from build123d import *

# Parameters (mm, degrees)
SKETCH1_W            = 105
SKETCH1_H            = 20
BOSS_EXTRUDE1_DEPTH  = 6.35
SKETCH3_W            = 23
SKETCH3_H            = 16
CUT_EXTRUDE1_DEPTH   = 54.819815124
SKETCH4_W            = 5
SKETCH4_H            = 12
CUT_EXTRUDE2_DEPTH   = 2
M2_CLEARANCE_HOLE1_D = 2


with BuildPart() as part:
    # Sketch1 → Boss-Extrude1 (new body)
    with BuildSketch(Plane(origin=(0, 0, 0), x_dir=(1, 0, 0), z_dir=(0, 1, 0))):
        Rectangle(SKETCH1_W, SKETCH1_H)
    extrude(amount=BOSS_EXTRUDE1_DEPTH)

    # Sketch3 → Cut-Extrude1 (cut, through all)
    with BuildSketch(Plane(origin=(0, 6.35, 0), x_dir=(1, 0, 0), z_dir=(0, 1, 0))):
        with Locations((-36, -2)):
            Rectangle(SKETCH3_W, SKETCH3_H)
        with Locations((36, 2)):
            Rectangle(SKETCH3_W, SKETCH3_H)
    extrude(amount=-CUT_EXTRUDE1_DEPTH, mode=Mode.SUBTRACT)

    # Sketch4 → Cut-Extrude2 (cut)
    with BuildSketch(Plane.XZ):
        with Locations((22, 0)):
            Rectangle(SKETCH4_W, SKETCH4_H)
        with Locations((50, 0)):
            Rectangle(SKETCH4_W, SKETCH4_H)
    extrude(amount=-CUT_EXTRUDE2_DEPTH, mode=Mode.SUBTRACT)

    # M2 Clearance Hole1 (through all)
    with Locations(Plane(origin=(0, 6.35, 0), x_dir=(1, 0, 0), z_dir=(0, 1, 0))):
        with Locations((50, 0), (-50, 0), (-22, 0), (22, 0)):
            Hole(M2_CLEARANCE_HOLE1_D / 2)


solid = part.part
Could you check a few things on this model? Use its own coordinates, in mm. A direction names the side the tool comes from. Round coordinates to 2 decimals unless told otherwise and drop trailing zeros. Write each loop counter-clockwise with the first axis right and the second up, starting at its lowest first coordinate (ties: lowest second). Pieces come first, ordered by that corner, then holes. Notation, with made-up numbers: (3, 57) - (19, 57) arc R29 ccw to (19, 81) - close; hole circle Ø4 at (39, 83). An arc over 180 degrees is marked (long way). Use a Markdown table: item, result.
Q1. For faces 1 (the flat face through (24.5, 4, -2)), 2 (the flat face through (-24.5, 3, 2)), 3 (the flat face through (48.85, 2, 0.08)), 4 (the flat face through (52.5, 4, 0)), which set-ups out of +Z, -Z, +X, -X, +Y, -Y let a thin tool reach every point of the face, with its end or its side?
Output values:
| item | result |
|---|---|
| face 1 | -Z, +Y, -Y |
| face 2 | +Z, +Y, -Y |
| face 3 | +X, -Y |
| face 4 | +Z, -Z, +X, +Y, -Y |
Q2. I want a section at B-B (x = 22). List the corners of the cut face in (y, z) for me, plus the area to 3 significant figures.
Output values:
| item | result |
|---|---|
| outline | (0, -10) - (6.35, -10) - (6.35, -1) - (2, -1) - (2, -6) - (0, -6) - close; (0, 6) - (2, 6) - (2, 1) - (6.35, 1) - (6.35, 10) - (0, 10) - close |
| area | 94.3 mm2 |
Q3. Thinking about a two-plate mould opening in X: for faces 5 (the flat face through (19.5, 1, 0)), 6 (the cylindrical face through (23, 4, 0)), 7 (the flat face through (-15, 3, -10)), which applies, released by +X, released by -X, zero draft, split by the parting line, or undercut?
Output values:
| item | result |
|---|---|
| face 5 | released by +X |
| face 6 | undercut |
| face 7 | zero draft |
Q4. I want a section at A-A (z = 0). Count the separate pieces of the cut face and the enclosed holes in it, plus the area to 3 significant figures.
Output values:
| item | result |
|---|---|
| separate pieces | 7 |
| enclosed holes | 0 |
| area | 312 mm2 |
Q5. For pin 1 (3 mm diameter, centred on x = 39.5, y = 4.5, fed in from -Z); pin 2 (1.8 mm diameter, centred on x = 50, z = 0, fed in from +Y); pin 3 (1 mm diameter, centred on y = 0.5, z = -1.5, fed in from +X); pin 4 (2.5 mm diameter, centred on x = 49.5, z = -1, fed in from -Y), each with a flat end and sliding along its axis, tell me the tip position at first contact or that it passes through.
Output values:
| item | result |
|---|---|
| pin 1 | z = 6 |
| pin 2 | through |
| pin 3 | x = 19.5 |
| pin 4 | y = 2 |
Q6. Please list where these lines run through material, in increasing order: L1, parallel to X at y = 4.75, z = -3.75; L2, parallel to X at y = 1, z = 6.5; L3, parallel to X at y = 0.75, z = 2.5.
Output values:
| item | result |
|---|---|
| L1 | -52.5 to -47.5, -24.5 to 24.5, 47.5 to 52.5 |
| L2 | -52.5 to -47.5, -24.5 to 52.5 |
| L3 | -52.5 to -47.5, -24.5 to 19.5 |
Q7. I want a section at D-D (y = 3.5). List the corners of the cut face in (x, z) for me, plus the area to 3 significant figures.
Output values:
| item | result |
|---|---|
| outline | (-52.5, -10) - (24.5, -10) - (24.5, 6) - (47.5, 6) - (47.5, -10) - (52.5, -10) - (52.5, 10) - (-24.5, 10) - (-24.5, -6) - (-47.5, -6) - (-47.5, 10) - (-52.5, 10) - close; hole circle Ø2 at (-50, 0); hole circle Ø2 at (-22, 0); hole circle Ø2 at (22, 0); hole circle Ø2 at (50, 0) |
| area | 1,350 mm2 |
Q8. I want a section at C-C (z = -7). List the corners of the cut face in (x, y) for me.
Output values:
| item | result |
|---|---|
| outline | (-52.5, 0) - (24.5, 0) - (24.5, 6.35) - (-52.5, 6.35) - close; (47.5, 0) - (52.5, 0) - (52.5, 6.35) - (47.5, 6.35) - close |
